from build123d import *

# Parameters (mm, degrees)
ESQUISSE1_R        = 2
ESQUISSE1_W        = 5
ESQUISSE1_H        = 10
BOSS_EXTRU_1_DEPTH = 6


with BuildPart() as part:
    # Esquisse1 → Boss.-Extru.1 (new body)
    with BuildSketch(Plane.XY):
        Polygon((0, 0), (0, 26), (-5.2, 26), (-5.2, 20), (-10, 20), (-10, 26), (-15.2, 26), (-15.2, 20), (-20, 20), (-20, 26), (-25.2, 26), (-25.2, 20), (-30, 20), (-30, 26), (-35.2, 26), (-35.2, 20), (-40, 20), (-40, 26), (-45.2, 26), (-45.2, 20), (-50, 20), (-50, 26), (-55.2, 26), (-55.2, 20), (-60, 20), (-60, 26), (-65.2, 26), (-65.2, 20), (-70, 20), (-70, 26), (-75.2, 26), (-75.2, 20), (-80, 20), (-80, 26), (-85.2, 26), (-85.2, 20), (-90, 20), (-90, 26), (-95.2, 26), (-95.2, 20), (-100, 20), (-100, 26), (-105.2, 26), (-105.2, 20), (-110, 20), (-110, 26), (-115.2, 26), (-115.2, 20), (-120, 20), (-120, 26), (-125.2, 26), (-125.2, 20), (-130, 20), (-130, 26), (-135.2, 26), (-135.2, 20), (-140, 20), (-140, 26), (-145.2, 26), (-145.2, 20), (-150, 20), (-150, 26), (-155.2, 26), (-155.2, 20), (-160, 20), (-160, 26), (-165.2, 26), (-165.2, 20), (-170, 20), (-170, 26), (-175.2, 26), (-175.2, 20), (-180, 20), (-180, 26), (-185.2, 26), (-185.2, 20), (-190, 20), (-190, 26), (-195.2, 26), (-195.2, 20), (-200, 20), (-200, 26), (-205.2, 26), (-205.2, 20), (-210, 20), (-210, 26), (-215.2, 26), (-215.2, 20), (-220, 20), (-220, 26), (-225.2, 26), (-225.2, 20), (-230, 20), (-230, 26), (-235.2, 26), (-235.2, 20), (-240, 20), (-240, 26), (-245.2, 26), (-245.2, 20), (-250, 20), (-250, 14.8), (-244, 14.8), (-244, 10), (-250, 10), (-250, 4.8), (-244, 4.8), (-244, 0), (-250, 0), (-250, -5.2), (-244, -5.2), (-244, -10), (-250, -10), (-250, -15.2), (-244, -15.2), (-244, -20), (-224, -20), (-224, 0), (-59.8, 0), (-59.8, 6), (-50, 6), (-50, 0), align=None)
        with Locations((-210, 10)):
            Circle(ESQUISSE1_R, mode=Mode.SUBTRACT)
        with Locations((-10, 10)):
            Circle(ESQUISSE1_R, mode=Mode.SUBTRACT)
        with Locations((-236.5, -5)):
            Rectangle(ESQUISSE1_W, ESQUISSE1_H, mode=Mode.SUBTRACT)
    extrude(amount=BOSS_EXTRU_1_DEPTH)


solid = part.part
Can you work these out from the model? Positions are in its coordinate system, mm. A direction names the side the tool comes from. Coordinates: 2 decimals unless noted, no trailing zeros. Write each loop counter-clockwise with the first axis right and the second up, starting at its lowest first coordinate (ties: lowest second). Pieces come first, ordered by that corner, then holes.
Q1. If we mould it in two halves opening along X, with no side actions, what happens to faces 4 (the face through (-105.2, 23, 3)), 5 (the face through (0, 13, 3)), 6 (the face through (-127, 14, 0))? For each: +X half, -X half, draft (parallel to the pull), parting line (faces both ways), or undercut.
Results found:
face 4: undercut
face 5: +X half
face 6: draft
Q2. Imagine slicing it at B-B, the plane z = 2.15. Count the separate pieces of the cut face and the enclosed holes in it, plus the area to 3 significant figures.
Results found:
separate pieces: 1
enclosed holes: 3
area: 6,050 mm2
Q3. Please list where these lines run through material, in increasing order: L1, parallel to Y at x = -227, z = 2.6; L2, parallel to X at y = 9, z = 2.45; L3, parallel to Y at x = -183, z = 0.25.
Results found:
L1: y = -20 to 20
L2: x = -250 to -211.73, -208.27 to -11.73, -8.27 to 0
L3: y = 0 to 26
Q4. Imagine slicing it at A-A, the plane x = -33. List the corners of the cut face in (y, z) for me.
Results found:
outline: (0, 0) - (26, 0) - (26, 6) - (0, 6) - close
Q5. For P1, Ø1.4, axis at x = -38, z = 4, coming from the +Y side; P2, Ø3, axis at y = 23.5, z = 4.5, coming from the -X side; P3, Ø3, axis at y = 2.5, z = 4.5, coming from the -X side, each with a flat end and sliding along its axis, tell me the tip position at first contact or that it passes through.
Results found:
P1: stops at y = 20
P2: stops at x = -245.2
P3: stops at x = -244
Q6. Which directions (+Z, -Z, +X, -X, +Y, -Y) give clear straight access to the entire face, cutting with the end or side of a thin tool? Please do faces 1 (the face through (-203, 26, 3)), 2 (the face through (-118, 20, 3)), 3 (the face through (-247, 4.8, 3)).
Results found:
face 1: +Z, -Z, +X, -X, +Y
face 2: +Z, -Z, +Y
face 3: +Z, -Z, -X
